from build123d import *

# Parameters (mm, degrees)
ESBO_O2_W                                    = 35
ESBO_O2_H                                    = 30
RESSALTO_EXTRUS_O1_DEPTH                     = 12
BROCA_DE_ROSQUEAR_PARA_TARRAXA_DE_M5X0_8_D   = 4.2
BROCA_DE_ROSQUEAR_PARA_TARRAXA_DE_M5_2_D     = 4.2
BROCA_DE_ROSQUEAR_PARA_TARRAXA_DE_M5_2_DEPTH = 20
BROCA_DE_ROSQUEAR_PARA_TARRAXA_DE_M5_2_TIP   = 1.2618073
CHANFRO1_SIZE                                = 1.5
CHANFRO2_SIZE                                = 1.5
CHANFRO3_SIZE                                = 1.5


with BuildPart() as part:
    # Esboço2 → Ressalto-extrusão1 (new body)
    with BuildSketch(Plane.XY):
        with Locations((119.430382681, 3.163019551)):
            Rectangle(ESBO_O2_W, ESBO_O2_H)
    extrude(amount=RESSALTO_EXTRUS_O1_DEPTH)

    # Broca de rosquear para tarraxa de M5x0.8 (through all)
    with Locations(Plane.XY.offset(12)):
        with Locations((111.330382681, 13.163019551), (111.330382681, 1.163019551)):
            Hole(BROCA_DE_ROSQUEAR_PARA_TARRAXA_DE_M5X0_8_D / 2)

    # Broca de rosquear para tarraxa de M5 2
    with Locations(Plane.XZ.offset(11.836980449)):
        with Locations((130.930382681, 6)):
            Hole(BROCA_DE_ROSQUEAR_PARA_TARRAXA_DE_M5_2_D / 2, depth=BROCA_DE_ROSQUEAR_PARA_TARRAXA_DE_M5_2_DEPTH)
            with Locations((0, 0, -(BROCA_DE_ROSQUEAR_PARA_TARRAXA_DE_M5_2_DEPTH + BROCA_DE_ROSQUEAR_PARA_TARRAXA_DE_M5_2_TIP / 2))):  # 118° drill point
                Cone(0, BROCA_DE_ROSQUEAR_PARA_TARRAXA_DE_M5_2_D / 2, BROCA_DE_ROSQUEAR_PARA_TARRAXA_DE_M5_2_TIP, mode=Mode.SUBTRACT)

    # Chanfro1
    chanfro1_edges = [part.edges().sort_by_distance(p)[0] for p in [
        (113.430382681, 1.163019551, 12),
        (113.430382681, 13.163019551, 12),
    ]]
    chamfer(chanfro1_edges, length=CHANFRO1_SIZE)

    # Chanfro2
    chanfro2_edges = [part.edges().sort_by_distance(p)[0] for p in [
        (113.430382681, 1.163019551, 0),
    ]]
    chamfer(chanfro2_edges, length=CHANFRO2_SIZE)

    # Chanfro3
    chanfro3_edges = [part.edges().sort_by_distance(p)[0] for p in [
        (113.430382681, 13.163019551, 0),
    ]]
    chamfer(chanfro3_edges, length=CHANFRO3_SIZE)


solid = part.part
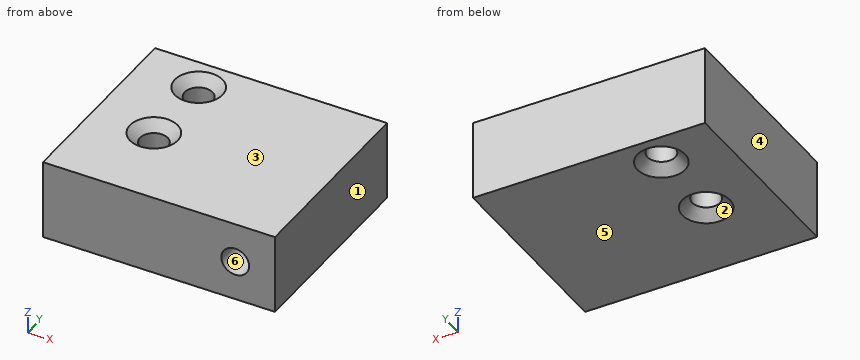
Part model, mm, in its own coordinate system. Face numbers are marked on the shaded views. A direction names the side the tool comes from. Round coordinates to 2 decimals unless told otherwise and drop trailing zeros. Write each loop counter-clockwise with the first axis right and the second up, starting at its lowest first coordinate (ties: lowest second). Pieces come first, ordered by that corner, then holes. Notation, with made-up numbers: M 26,41 L 34,41 A17 cw 34,50 Z; hole C 23,67 d11. An arc over 180 degrees is marked long. Return JSON: item names as keys, results as strings. Group by question number.
(1) Saw through at C-C on y = 0. Count the separate pieces of the cut face and the enclosed holes in it, then the cut area to 3 significant figures.
(2) Saw through at B-B on z = 2.5. Write the cut outline in (x, y), then the cut area to 3 significant figures.
(3) Which spindle directions (+Z, -Z, +X, -X, +Y, -Y) get a long thin tool onto all of the face, cutting with end or side? Do the marked faces 5 and 6. Say none if no direction does.
(4) Two-plate mould, pull along X, no slides. Class the marked faces 1, 2, 3 and 4: +X half, -X half, draft (parallel to the pull), parting line (faces both ways), or undercut.
(5) Pin check, flat tip, straight feed: pin 1 Ø1 at (x, y) = (109.5, -1.5) entering from -Z. Stop position of the tip, or through.
(6) Drill centre lines: probe 1 along Y at (x, z) = (111.5, 8.5); probe 2 along X at (y, z) = (-6, 6); probe 3 along X at (y, z) = (1, 6.5). Where is each one in solid material? Low to high.
(7) Saw through at A-A on y = 7. Write the cut outline in (x, z), then the cut area to 3 significant figures.
(8) Saw through at D-D on z = 11. Write the cut outline in (x, y), then the cut area to 3 significant figures.
Returned:
{
 "1": {"separate pieces": "2", "enclosed holes": "1", "area": "359 mm²"},
 "2": {"outline": "M 101.93,-11.84 L 136.93,-11.84 L 136.93,18.16 L 101.93,18.16 Z; hole C 111.33,1.16 d4.2; hole C 111.33,13.16 d4.2", "area": "1,020 mm²"},
 "3": {"face 5": "-Z, +X, -X, +Y, -Y", "face 6": "-Y"},
 "4": {"face 1": "+X half", "face 2": "undercut", "face 3": "draft", "face 4": "-X half"},
 "5": {"pin 1": "z = 0"},
 "6": {"probe 1": "-11.84 to -0.93, 3.26 to 11.07, 15.26 to 18.16", "probe 2": "101.93 to 128.83, 133.03 to 136.93", "probe 3": "101.93 to 109.24, 113.42 to 128.89, 132.97 to 136.93"},
 "7": {"outline": "M 101.93,0 L 136.93,0 L 136.93,12 L 101.93,12 Z; hole C 130.93,6 d4.2", "area": "406 mm²"},
 "8": {"outline": "M 101.93,-11.84 L 136.93,-11.84 L 136.93,18.16 L 101.93,18.16 Z; hole C 111.33,1.16 d5.2; hole C 111.33,13.16 d5.2", "area": "1,010 mm²"}
}
